Can you work these out from the model? Positions are in its coordinate system, mm. A direction names the side the tool comes from. Give positions to 0.01 mm unless a question says otherwise; leave off trailing zeros. Write each loop counter-clockwise with the first axis right and the second up, starting at its lowest first coordinate (ties: lowest second). Pieces come first, ordered by that corner, then holes. Notation, with made-up numbers: M 62.5,-14 L 106.5,-14 A30 ccw 106.5,13 Z; hole C -35.75,41 d11. An arc over 180 degrees is marked long. Write each question's results on one line, items separated by ' | '.
from build123d import *

# Parameters (mm, degrees)
SKETCH1_R           = 2.75
BOSS_EXTRUDE1_DEPTH = 15
SKETCH2_R           = 2
CUT_EXTRUDE1_DEPTH  = 41
SKETCH3_R           = 4.5
CUT_EXTRUDE2_DEPTH  = 5
SKETCH4_R           = 4.5
CUT_EXTRUDE3_DEPTH  = 5
CUT_EXTRUDE4_REACH  = 37
SKETCH5_R           = 2.75


with BuildPart() as part:
    # Sketch1 → Boss-Extrude1 (new body)
    with BuildSketch(Plane.XY):
        with BuildLine():
            Line((0, 0), (100, 0))
            Line((100, 0), (100, 17))
            Line((100, 17), (64.696938457, 17))
            ThreePointArc((64.696938457, 17), (50, 5), (35.303061543, 17))
            Line((35.303061543, 17), (20, 17))
            ThreePointArc((20, 17), (17, 20), (20, 23))
            Line((20, 23), (35.303061543, 23))
            ThreePointArc((35.303061543, 23), (50, 35), (64.696938457, 23))
            Line((64.696938457, 23), (100, 23))
            Line((100, 23), (100, 40))
            Line((100, 40), (0, 40))
            Line((0, 40), (0, 0))
        make_face()
        with Locations((10, 30)):
            Circle(SKETCH1_R, mode=Mode.SUBTRACT)
        with Locations((10, 10)):
            Circle(SKETCH1_R, mode=Mode.SUBTRACT)
        with Locations((90, 30)):
            Circle(SKETCH1_R, mode=Mode.SUBTRACT)
    extrude(amount=BOSS_EXTRUDE1_DEPTH)

    # Sketch2 → Cut-Extrude1 (cut, through all)
    with BuildSketch(Plane.XZ):
        with Locations((75, 7.5)):
            Circle(SKETCH2_R)
    extrude(amount=-CUT_EXTRUDE1_DEPTH, mode=Mode.SUBTRACT)

    # Sketch3 → Cut-Extrude2 (cut)
    with BuildSketch(Plane.XZ):
        with Locations((75, 7.5)):
            Circle(SKETCH3_R)
    extrude(amount=-CUT_EXTRUDE2_DEPTH, mode=Mode.SUBTRACT)

    # Sketch4 → Cut-Extrude3 (cut)
    with BuildSketch(Plane.XY):
        with Locations((10, 10)):
            Circle(SKETCH4_R)
        with Locations((10, 30)):
            Circle(SKETCH4_R)
        with Locations((90, 30)):
            Circle(SKETCH4_R)
    extrude(amount=CUT_EXTRUDE3_DEPTH, mode=Mode.SUBTRACT)

    # Sketch5 → Cut-Extrude4 (cut, up to next)
    with BuildSketch(Plane.XZ.offset(-5), mode=Mode.PRIVATE) as cut_extrude4_sk1:
        with Locations((75, 7.5)):
            Circle(SKETCH5_R)
    cut_extrude4_tool1 = extrude(cut_extrude4_sk1.sketch, amount=-CUT_EXTRUDE4_REACH, mode=Mode.PRIVATE) & part.part
    add(cut_extrude4_tool1.solids().sort_by_distance((75, 5, 7.5))[0], mode=Mode.SUBTRACT)


solid = part.part
Item 1: If I drill on line 1 (Y direction, x = 10, z = 12.75); line 2 (Z direction, x = 75, y = 3.85); line 3 (Y direction, x = 77, z = 3.75), over which ranges is the centre line in solid material (lowest first)? Write a range as from..to.
Geometry says:
line 1: y = 0..7.25, 12.75..27.25, 32.75..40 | line 2: z = 0..3, 12..15 | line 3: y = 5..17, 23..40
Item 2: I want a section at D-D, the plane y = 30. Please give me the cut outline in (x, z).
Geometry says:
outline: M 0,0 L 5.5,0 L 5.5,5 L 7.25,5 L 7.25,15 L 0,15 Z; M 12.75,5 L 14.5,5 L 14.5,0 L 38.82,0 L 38.82,15 L 12.75,15 Z; M 61.18,0 L 85.5,0 L 85.5,5 L 87.25,5 L 87.25,15 L 61.18,15 Z; M 92.75,5 L 94.5,5 L 94.5,0 L 100,0 L 100,15 L 92.75,15 Z; hole C 75,7.5 d4
Item 3: I want a section at A-A, the plane z = 7.5. Please give me the cut outline in (x, y), and give its area (3 significant figures).
Geometry says:
outline: M 0,0 L 70.5,0 L 70.5,5 L 72.25,5 L 72.25,17 L 64.7,17 A15 cw 35.3,17 L 20,17 A3 cw 20,23 L 35.3,23 A15 cw 64.7,23 L 73,23 L 73,40 L 0,40 Z; M 77,23 L 100,23 L 100,40 L 77,40 Z; M 77.75,5 L 79.5,5 L 79.5,0 L 100,0 L 100,17 L 77.75,17 Z; hole C 10,10 d5.5; hole C 10,30 d5.5; hole C 90,30 d5.5 | area: 2,730 mm2
Item 4: I want a section at C-C, the plane y = 10. Please give me the cut outline in (x, z), and give its area (3 significant figures).
Geometry says:
outline: M 0,0 L 5.5,0 L 5.5,5 L 7.25,5 L 7.25,15 L 0,15 Z; M 12.75,5 L 14.5,5 L 14.5,0 L 38.82,0 L 38.82,15 L 12.75,15 Z; M 61.18,0 L 100,0 L 100,15 L 61.18,15 Z; hole C 75,7.5 d5.5 | area: 1,040 mm2
Item 5: I'm going to push flat-ended pins straight in: pin 1 (14.5 mm diameter, centred on x = 90, y = 30, fed in from -Z); pin 2 (2.5 mm diameter, centred on x = 89, y = 31.5, fed in from -Z); pin 3 (5 mm diameter, centred on x = 75, z = 7.5, fed in from -Y); pin 4 (3.5 mm diameter, centred on x = 75, z = 7.5, fed in from -Y). Where does each tip first touch, or does it pass through?
Geometry says:
pin 1: stops at z = 0 | pin 2: stops at z = 5 | pin 3: stops at y = 23 | pin 4: passes through
Item 6: For faces 5 (the face through (14.292, 11.352, 2.465)), 6 (the face through (50, 5, 7)), 7 (the face through (72.253, 10.916, 7.621)), which set-ups out of +Z, -Z, +X, -X, +Y, -Y let a thin tool reach every point of the face, with its end or its side?
Geometry says:
face 5: -Z | face 6: +Z, -Z | face 7: -Y
Item 7: Thinking about a two-plate mould opening in X: for faces 1 (the face through (13, 30, 5)), 2 (the face through (10, 7, 5)), 3 (the face through (82, 23, 7)), 4 (the face through (17, 20, 7)), which applies, +X half, -X half, draft (parallel to the pull), parting line (faces both ways), or undercut?
Geometry says:
face 1: undercut | face 2: undercut | face 3: draft | face 4: +X half
Item 8: I want a section at B-B, the plane x = 90. Please give me the cut outline in (y, z).
Geometry says:
outline: M 0,0 L 17,0 L 17,15 L 0,15 Z; M 23,0 L 25.5,0 L 25.5,5 L 27.25,5 L 27.25,15 L 23,15 Z; M 32.75,5 L 34.5,5 L 34.5,0 L 40,0 L 40,15 L 32.75,15 Z
